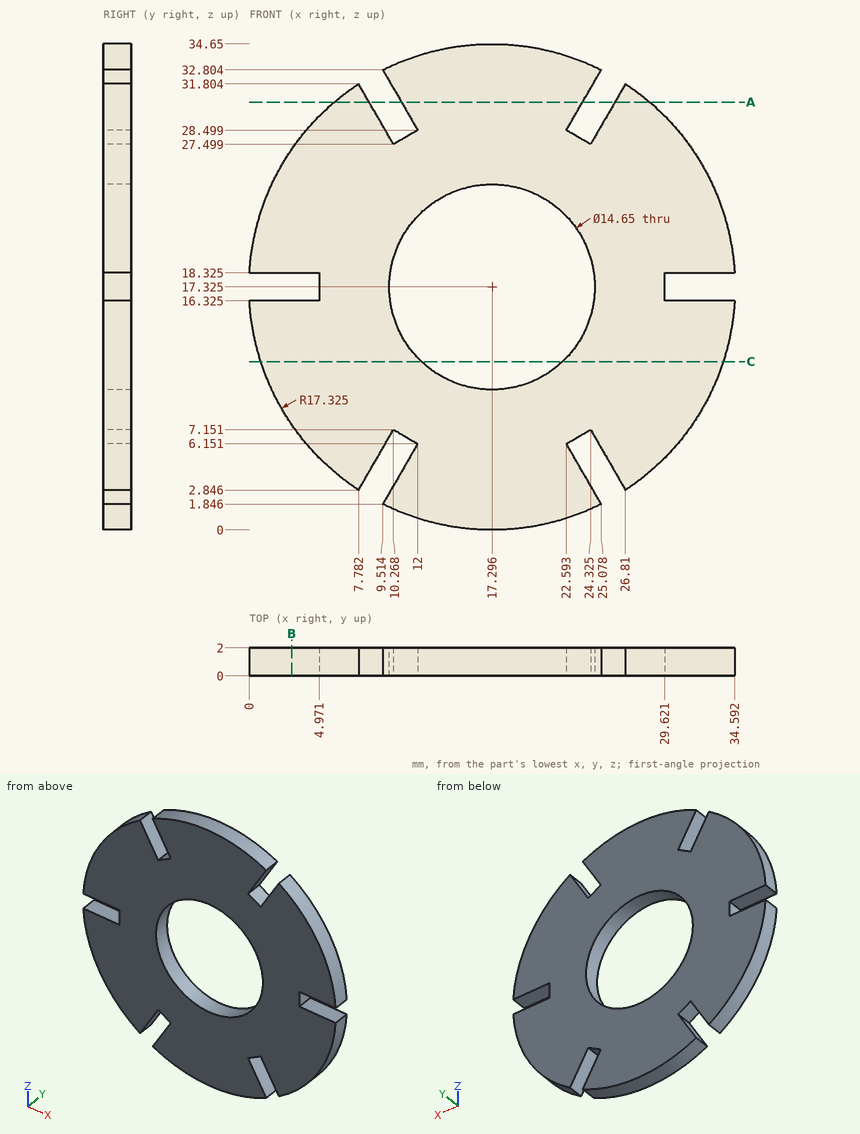
Print and shaded views of the part. All mm, measured from the part's lowest x, y and z. Coordinates: 2 decimals unless noted, no trailing zeros. Loops run counter-clockwise (first coordinate to the right, second up) from the corner with the lowest first, then second, coordinate; pieces in that order, holes last. Notation, with made-up numbers: (50.5, 35) -> (54.5, 35) arc R34 ccw to (54.5, 74) -> close; hole circle Ø8 at (17.25, 38.5). An arc over 180 degrees is marked (long way). Use a Markdown table: item, result. Add a question column.
Item 1: Band-saw the part on A-A on z = 30.5. Write the cut outline in (x, y) (1 decimal).
Item 2: Band-saw the part on C-C on z = 12. Write the cut outline in (x, y).
Item 3: Probe probe 1 along Z at (x, y) = (33, 1.4) (1 decimal); probe 2 along X at (y, z) = (0.85, 31) (1 decimal); probe 3 along X at (y, z) = (1.15, 7) (1 decimal). List the from-to ranges inside material, lowest first.
Item 4: Band-saw the part on B-B on x = 3. Write the cut outline in (y, z) (1 decimal).
Item 5: Flat gauge pins, fed straight in: P1, Ø1, axis at x = 32.5, y = 1, coming from the -Z side; P2, Ø0.6, axis at x = 1.5, y = 1.5, coming from the +Z side (1 decimal); P3, Ø1, axis at y = 1.5, z = 17.5, coming from the -X side. Where does each tip first touch, or does it go through?
Geometry says:
| question | item | result |
|---|---|---|
| 1 | outline | (6, 0) -> (8.5, 0) -> (8.5, 2) -> (6, 2) -> close; (10.8, 0) -> (23.7, 0) -> (23.7, 2) -> (10.8, 2) -> close; (26.1, 0) -> (28.5, 0) -> (28.5, 2) -> (26.1, 2) -> close |
| 2 | outline | (0.81, 0) -> (12.27, 0) -> (12.27, 2) -> (0.81, 2) -> close; (22.33, 0) -> (33.78, 0) -> (33.78, 2) -> (22.33, 2) -> close |
| 3 | probe 1 | 10 to 16.3, 18.3 to 24.6 |
| 3 | probe 2 | 6.7 to 8.2, 10.6 to 24, 26.3 to 27.9 |
| 3 | probe 3 | 3.4 to 10.2, 10.5 to 24.1, 24.4 to 31.2 |
| 4 | outline | (0, 7.5) -> (2, 7.5) -> (2, 16.3) -> (0, 16.3) -> close; (0, 18.3) -> (2, 18.3) -> (2, 27.1) -> (0, 27.1) -> close |
| 5 | P1 | z = 8.16 |
| 5 | P2 | z = 25.1 |
| 5 | P3 | x = 4.97 |
